Design review of the part built by this model. Coordinates are the model's own, in mm. Coordinates: 2 decimals unless noted, no trailing zeros. Loops run counter-clockwise (first coordinate to the right, second up) from the corner with the lowest first, then second, coordinate; pieces in that order, holes last.
from build123d import *

# Parameters (mm, degrees)
BOSS_EXTRUDE1_DEPTH = 1.5
BOSS_EXTRUDE1_DRAFT = 20
FILLET1_R           = 1


with BuildPart() as part:
    # Sketch1 → Boss-Extrude1 (with draft: the straight prism first)
    with BuildSketch(Plane(origin=(0, 0, 0), x_dir=(1, 0, 0), z_dir=(0, 1, 0))):
        with BuildLine():
            Line((2.105043255, 5.618611296), (0, 19.137920482))
            Line((0, 19.137920482), (-2.105043255, 5.618611296))
            ThreePointArc((-2.105043255, 5.618611296), (-6, 0), (-2.105043255, -5.618611296))
            Line((-2.105043255, -5.618611296), (0, -19.137920482))
            Line((0, -19.137920482), (2.105043255, -5.618611296))
            ThreePointArc((2.105043255, -5.618611296), (6, 0), (2.105043255, 5.618611296))
        make_face()
    extrude(amount=BOSS_EXTRUDE1_DEPTH)
    # Boss-Extrude1: the draft: its side faces are tilted about the plane it starts from
    boss_extrude1_sides = [part.faces().sort_by_distance(p)[0] for p in [
        (1.052521627, 0.75, -12.378265889),
        (-1.052521627, 0.75, -12.378265889),
        (-6, 0.75, 0),
        (-1.052521627, 0.75, 12.378265889),
        (1.052521627, 0.75, 12.378265889),
        (6, 0.75, 0),
    ]]
    draft(boss_extrude1_sides, Plane(origin=(0, 0, 0), x_dir=(1, 0, 0), z_dir=(0, 1, 0)), BOSS_EXTRUDE1_DRAFT)

    # Fillet1
    fillet1_edges = [part.edges().sort_by_distance(p)[0] for p in [
        (-0.80814003, 1.5, 10.399206057),
        (-5.454044649, 1.5, 0),
        (-0.80814003, 1.5, -10.399206057),
        (0.80814003, 1.5, -10.399206057),
        (5.454044649, 1.5, 0),
        (0.80814003, 1.5, 10.399206057),
    ]]
    fillet(fillet1_edges, radius=FILLET1_R)


solid = part.part
Q1. For line 1 (Z direction, x = -2, y = 1.2); line 2 (X direction, y = 0.8, z = 1.5); line 3 (X direction, y = 1.15, z = 7), list the stretches that pass through material, from the lowest coordinate up.
Q2. Take a section at A-A, the plane y = 0.35. Write out the cut boundary in (x, z).
Q3. Clearance check with a flat-ended pin moving along its axis: pin 1 Ø4 at (x, z) = (3.5, -8) entering from -Y. State where the tip first meets the part, or that it passes through.
Entries:
1. line 1: z = -5.09 to 5.09
1. line 2: x = -5.51 to 5.51
1. line 3: x = -1.4 to 1.4
2. outline: (-1.99, -5.52) - (0, -18.31) - (1.99, -5.52) arc R5.87 ccw to (1.99, 5.52) - (0, 18.31) - (-1.99, 5.52) arc R5.87 ccw to start
3. pin 1: stops at y = 0
